Verification items for the finished model (mm, model axes). Face numbers are marked on the shaded views. A direction names the side the tool comes from. Round coordinates to 2 decimals unless told otherwise and drop trailing zeros. Write each loop counter-clockwise with the first axis right and the second up, starting at its lowest first coordinate (ties: lowest second). Pieces come first, ordered by that corner, then holes. Notation, with made-up numbers: (-35, 52) - (13, 52) arc R35 cw to (13, 89) - close; hole circle Ø1 at (-3, 83). An arc over 180 degrees is marked (long way). Write each question's results on one line, items separated by ' | '.
```python
from build123d import *

# Parameters (mm, degrees)
F1_DEPTH = 3.5
F2_DEPTH = 4.5
F3_DEPTH = 4
F4_W     = 1.984375
F4_H     = 1
F5_DEPTH = 25
F6_START = 1
F4_W_2   = 15.314116451
F4_H_2   = 5
F6_DEPTH = 2.96975


with BuildPart() as f1:
    # F0 (on Front) → F1 (new body, symmetric)
    with BuildSketch(Plane.XZ):
        with BuildLine():
            ThreePointArc((1.984375, 1.984375), (1.4031650189, 0.5812099811), (0, 0))
            Line((0, 0), (23.314116451, 0))
            ThreePointArc((23.314116451, 0), (22.1516964889, 2.8063300378), (19.345366451, 3.96875))
            Line((19.345366451, 3.96875), (0, 3.96875))
            ThreePointArc((0, 3.96875), (1.4031650189, 3.3875400189), (1.984375, 1.984375))
        make_face()
        with BuildLine():
            ThreePointArc((-1.9442824833, 1.5875), (-1.2550289464, 0.4472847345), (0, 0))
            ThreePointArc((0, 0), (1.4031650189, 0.5812099811), (1.984375, 1.984375))
            ThreePointArc((1.984375, 1.984375), (1.4031650189, 3.3875400189), (0, 3.96875))
            ThreePointArc((0, 3.96875), (-1.2550289464, 3.5214652655), (-1.9442824833, 2.38125))
            Line((-1.9442824833, 2.38125), (-1.1225320151, 2.38125))
            ThreePointArc((-1.1225320151, 2.38125), (0.2013370434, 3.1578532851), (1.190625, 1.984375))
            ThreePointArc((1.190625, 1.984375), (0.2013370434, 0.8108967149), (-1.1225320151, 1.5875))
            Line((-1.1225320151, 1.5875), (-1.9442824833, 1.5875))
        make_face()
        with BuildLine():
            ThreePointArc((-1.9442824833, 2.38125), (-1.984375, 1.984375), (-1.9442824833, 1.5875))
            Line((-1.9442824833, 1.5875), (-1.1225320151, 1.5875))
            ThreePointArc((-1.1225320151, 1.5875), (-1.190625, 1.984375), (-1.1225320151, 2.38125))
            Line((-1.1225320151, 2.38125), (-1.9442824833, 2.38125))
        make_face()
    extrude(amount=F1_DEPTH, both=True)

    # F0 (on Front) → F2 (join, symmetric)
    with BuildSketch(Plane.XZ):
        with BuildLine():
            ThreePointArc((-1.1225320151, 2.38125), (-1.190625, 1.984375), (-1.1225320151, 1.5875))
            ThreePointArc((-1.1225320151, 1.5875), (0.2013370434, 0.8108967149), (1.190625, 1.984375))
            ThreePointArc((1.190625, 1.984375), (0.2013370434, 3.1578532851), (-1.1225320151, 2.38125))
        make_face()
    extrude(amount=F2_DEPTH, both=True)

    # F0 (on Front) → F3 (join, symmetric)
    with BuildSketch(Plane.XZ):
        with BuildLine():
            ThreePointArc((-1.9442824833, 2.38125), (-1.984375, 1.984375), (-1.9442824833, 1.5875))
            Line((-1.9442824833, 1.5875), (-1.1225320151, 1.5875))
            ThreePointArc((-1.1225320151, 1.5875), (-1.190625, 1.984375), (-1.1225320151, 2.38125))
            Line((-1.1225320151, 2.38125), (-1.9442824833, 2.38125))
        make_face()
    extrude(amount=F3_DEPTH, both=True)

    # F4 (on Top) → F5 (cut)
    with BuildSketch(Plane.XY):
        with Locations((-0.9921875, 2)):
            Rectangle(F4_W, F4_H)
        with BuildLine():
            Line((0, 2.5), (0, 1.5))
            Line((0, 1.5), (2.515625, 1.5))
            ThreePointArc((2.515625, 1.5), (3.015625, 2), (2.515625, 2.5))
            Line((2.515625, 2.5), (0, 2.5))
        make_face()
        with Locations((-0.9921875, -2)):
            Rectangle(F4_W, F4_H)
        with BuildLine():
            Line((0, -1.5), (0, -2.5))
            Line((0, -2.5), (2.515625, -2.5))
            ThreePointArc((2.515625, -2.5), (3.015625, -2), (2.515625, -1.5))
            Line((2.515625, -1.5), (0, -1.5))
        make_face()
    extrude(amount=F5_DEPTH, mode=Mode.SUBTRACT)

    # F4 (on Top) → F6 (cut)
    with BuildSketch(Plane.XY.offset(F6_START)):
        with BuildLine():
            ThreePointArc((2.515625, -1.5), (3.015625, -2), (2.515625, -2.5))
            Line((2.515625, -2.5), (7.5, -2.5))
            Line((7.5, -2.5), (7.5, 2.5))
            Line((7.5, 2.5), (2.515625, 2.5))
            ThreePointArc((2.515625, 2.5), (3.015625, 2), (2.515625, 1.5))
            Line((2.515625, 1.5), (0, 1.5))
            Line((0, 1.5), (0, -1.5))
            Line((0, -1.5), (2.515625, -1.5))
        make_face()
        with Locations((15.6570582255, 0)):
            Rectangle(F4_W_2, F4_H_2)
    extrude(amount=F6_DEPTH, mode=Mode.SUBTRACT)


solid = f1.part
```
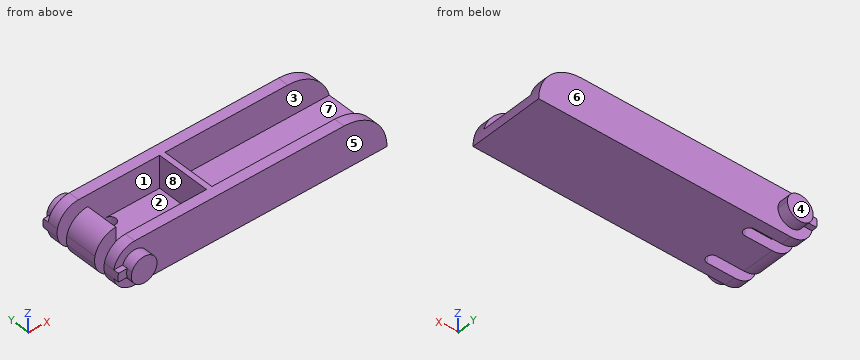
(1) Go/stop test with flat-tipped pins: pin 1 Ø1.5 at (y, z) = (1, 2.5) entering from +X; pin 2 Ø1.5 at (y, z) = (0, 3) entering from -X; pin 3 Ø1.5 at (x, z) = (18, 2) entering from +Y. Record where each tip stops, or that it passes through.
Answer:
pin 1: x = 8 | pin 2: x = -1.97 | pin 3: y = 3.5
(2) Thickness scan on L1, parallel to Y at x = 21, z = 2.9; L2, parallel to X at y = -1, z = 1.85; L3, parallel to Z at x = 18.25, y = 0.25. Record the ranges inside material, lowest first.
Answer:
L1: -3.5 to -2.5, 2.5 to 3.5 | L2: -1.98 to 0, 7.5 to 8 | L3: 0 to 1
(3) Mould release check, pull along Y, two halves, no side actions. Record for the marked faces 5, 6, 7 and 8: released by +Y, released by -Y, zero draft, split by the parting line, or undercut.
Answer:
face 5: released by -Y | face 6: released by +Y | face 7: undercut | face 8: undercut
(4) Section check C-C (y = -0.25). Record the cut outline in (x, z).
Answer:
outline: (0, 0) - (23.31, 0) arc R3.97 ccw to (23.19, 1) - (8, 1) - (8, 3.97) - (7.5, 3.97) - (7.5, 1) - (0, 1) - (0, 3.97) arc R1.98 ccw to start
(5) Section check A-A (y = 2). Record the cut outline in (x, z).
Answer:
outline: (3.02, 0) - (23.31, 0) arc R3.97 ccw to (23.19, 1) - (8, 1) - (8, 3.97) - (7.5, 3.97) - (7.5, 1) - (3.02, 1) - close
(6) Set-up check for the marked faces 1, 2, 3 and 4: record each of +Z, -Z, +X, -X, +Y, -Y from which the full face is reachable in a straight line by a thin tool's end or side.
Answer:
face 1: +Z, -X | face 2: +Z | face 3: +Z, +X | face 4: +Z, -Z, +X, -X, +Y
(7) Section check B-B (x = 13.5). Record the cut outline in (y, z).
Answer:
outline: (-3.5, 0) - (3.5, 0) - (3.5, 3.97) - (2.5, 3.97) - (2.5, 1) - (-2.5, 1) - (-2.5, 3.97) - (-3.5, 3.97) - close
